Design review of the part shown in the three views and the two pictorial views. Dimensions are in mm from the part's minimum x, y and z. Round coordinates to 2 decimals unless told otherwise and drop trailing zeros. Order: outer loops, then holes, each group sorted by start corner. A loop starts at its lowest first (then second) coordinate and runs counter-clockwise, first axis right, second up. Notation, with made-up numbers: (30, 53) -> (76, 53) arc R21 ccw to (76, 60) -> close; hole circle Ø4 at (-6, 89). An arc over 180 degrees is marked (long way). Put each result on its own line as item: value. Start each with the question number.
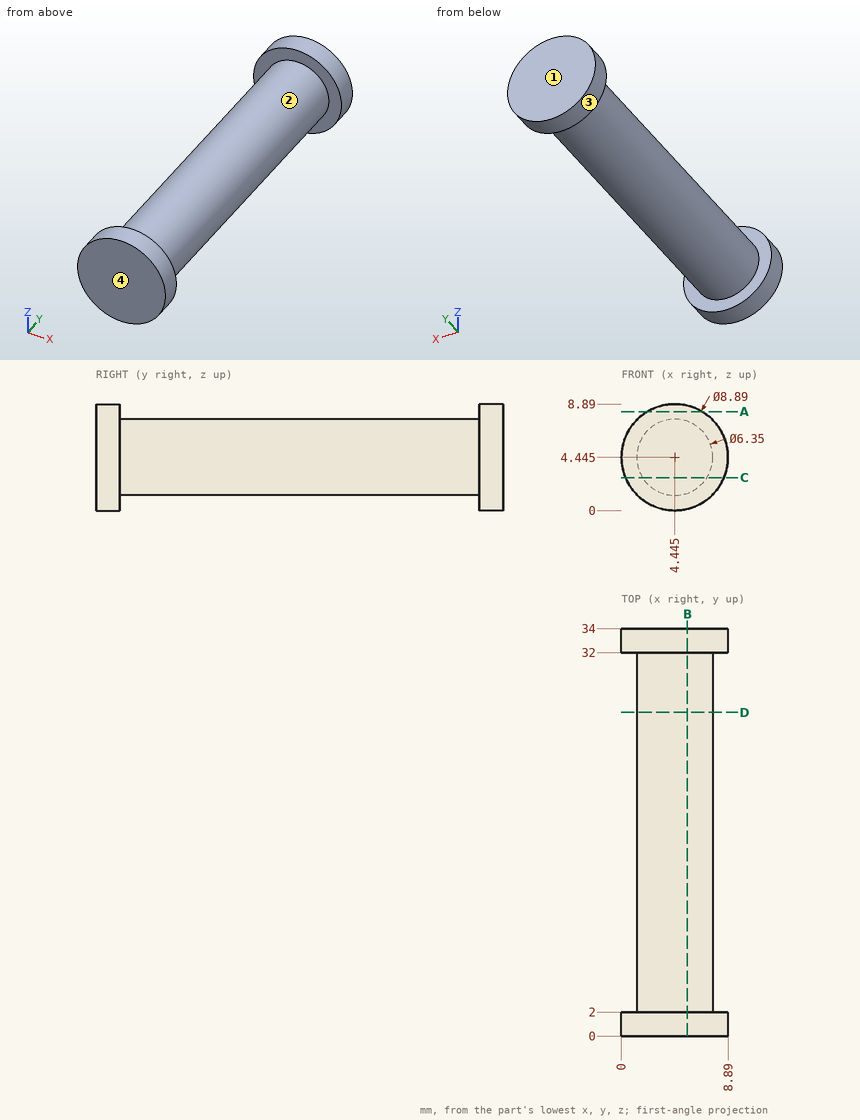
Q1. Take a section at D-D on y = 27. Give the boundary of the cut face in (x, z) (3 decimals).
Q2. Clearance check with flat-ended pins moving along their axes: pin 1 Ø1.5 at (y, z) = (16.5, 4.5) entering from +X; pin 2 Ø1 at (y, z) = (18, 3) entering from -X; pin 3 Ø1 at (x, z) = (6, 5.5) entering from -Y; pin 4 Ø4 at (y, z) = (22, 5) entering from -X. State where each tip first meets the part, or that it passes through.
Q3. Wall thickness on probe 1 along Y at (x, z) = (6.5, 8.25); probe 2 along X at (y, z) = (25, 4.25); probe 3 along Z at (x, y) = (2.25, 5): over which ranges is each line inside the solid? List them lowest first. Write a range as [from, to].
Q4. Take a section at B-B on x = 5.5. Give the boundary of the cut face in (y, z).
Q5. Draft analysis for pull direction Y (two halves, no side actions). For the marked faces 1, 2, 3 and 4, state which applies: +Y half, -Y half, draft (parallel to the pull), parting line (faces both ways), or undercut.
Q6. Take a section at C-C on z = 2.75. Give the boundary of the cut face in (x, y), and give its area (3 significant figures).
Q7. Take a section at A-A on z = 8.25. Give the boundary of the cut face in (x, y).
Calculated:
1. outline: circle Ø6.35 at (4.445, 4.445)
2. pin 1: stops at x = 7.62
2. pin 2: stops at x = 1.41
2. pin 3: stops at y = 0
2. pin 4: stops at x = 1.27
3. probe 1: y = [0, 2], [32, 34]
3. probe 2: x = [1.28, 7.61]
3. probe 3: z = [2.15, 6.74]
4. outline: (0, 0.13) -> (2, 0.13) -> (2, 1.45) -> (32, 1.45) -> (32, 0.13) -> (34, 0.13) -> (34, 8.76) -> (32, 8.76) -> (32, 7.44) -> (2, 7.44) -> (2, 8.76) -> (0, 8.76) -> close
5. face 1: +Y half
5. face 2: undercut
5. face 3: draft
5. face 4: -Y half
6. outline: (0.34, 0) -> (8.55, 0) -> (8.55, 2) -> (7.13, 2) -> (7.13, 32) -> (8.55, 32) -> (8.55, 34) -> (0.34, 34) -> (0.34, 32) -> (1.76, 32) -> (1.76, 2) -> (0.34, 2) -> close
6. area: 194 mm²
7. outline: (2.15, 0) -> (6.74, 0) -> (6.74, 2) -> (2.15, 2) -> close; (2.15, 32) -> (6.74, 32) -> (6.74, 34) -> (2.15, 34) -> close
